Can you work these out from the drawing? Everything is in mm from the part's minimum corner. Round coordinates to 2 decimals unless told otherwise and drop trailing zeros. Write each loop counter-clockwise with the first axis right and the second up, starting at its lowest first coordinate (ties: lowest second). Pieces come first, ordered by that corner, then holes. Notation, with made-up numbers: (74, 65.5) -> (96, 65.5) arc R30 ccw to (96, 101.5) -> close; hole circle Ø8 at (-21.75, 1). An arc over 180 degrees is marked (long way). Answer as CSV lines item,"result". Start each with the question number.
Q1. Imagine slicing it at B-B on y = 141.5. Please give me the cut outline in (x, z), and give its area (3 significant figures).
Q2. Imagine slicing it at A-A on x = 397. Please give me the cut outline in (y, z), and give its area (3 significant figures).
Q3. If I drill on line 1 (Y direction, x = 312.5, z = 5.5); line 2 (Y direction, x = 397, z = 14); line 3 (X direction, y = 139, z = 15), over which ranges is the centre line in solid material (lowest first)? Write a range as [from, to].
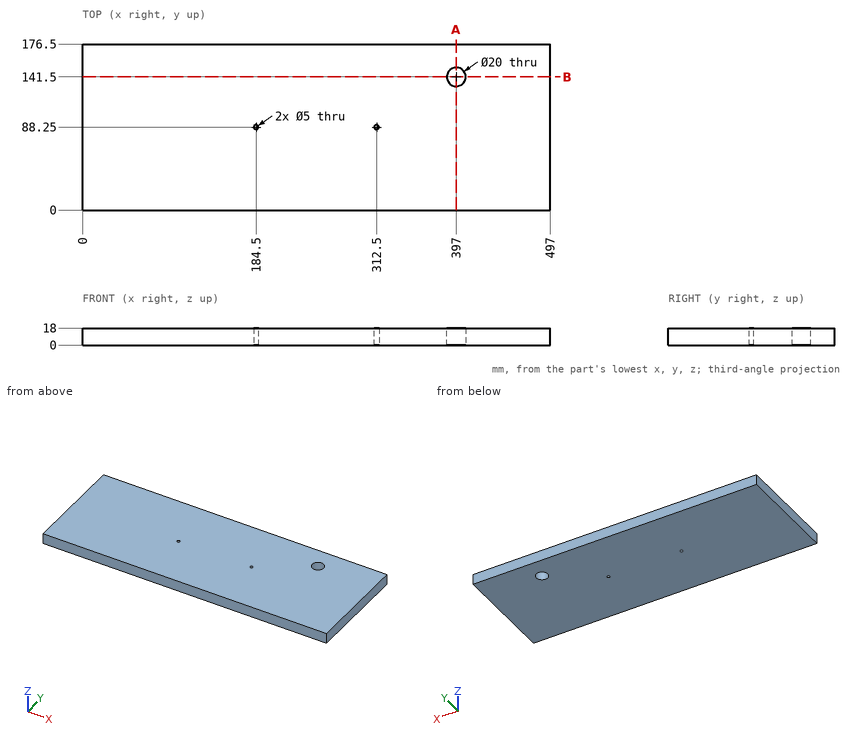
Checks:
1,outline,"(0, 0) -> (387, 0) -> (387, 18) -> (0, 18) -> close; (407, 0) -> (497, 0) -> (497, 18) -> (407, 18) -> close"
1,area,"8,590 mm^2"
2,outline,"(0, 0) -> (131.5, 0) -> (131.5, 18) -> (0, 18) -> close; (151.5, 0) -> (176.5, 0) -> (176.5, 18) -> (151.5, 18) -> close"
2,area,"2,820 mm^2"
3,line 1,"[0, 85.75], [90.75, 176.5]"
3,line 2,"[0, 131.5], [151.5, 176.5]"
3,line 3,"[0, 387.32], [406.68, 497]"
